```python
from build123d import *

# Parameters (mm, degrees)
HEX_START      = -10
SKETCH3_R      = 2
HEX_HEAD_DEPTH = 10


with BuildPart() as part:
    # Sketch1 → Main Base (revolve)
    with BuildSketch(Plane(origin=(0, 0, 0), x_dir=(0, 0, -1), z_dir=(1, 0, 0))):
        Polygon((0, 2), (0, 3), (-8.5, 3), (-8.5, 3.2), (-9.3, 4), (-14.2, 4), (-15, 3.2), (-17, 3.2), (-17, 5.9), (-18.6, 5.9), (-18.6, 7), (-28.6, 7), (-28.6, 2), align=None)
    revolve(axis=Axis((0, 0, -105.38083184), (0, 0, 1)))

    # Sketch3 → Hex Head (add)
    with BuildSketch(Plane.XY.offset(28.6).offset(HEX_START)):
        Polygon((8.082903769, 0), (4.041451884, 7), (-4.041451884, 7), (-8.082903769, 0), (-4.041451884, -7), (4.041451884, -7), align=None)
        with Locations(Location((0, 0, 0), (0, 0, 90))):
            Circle(SKETCH3_R, mode=Mode.SUBTRACT)
    extrude(amount=HEX_HEAD_DEPTH)

    # Sketch5 → Hex Trim (revolve, cut)
    with BuildSketch(Plane(origin=(0, 0, 0), x_dir=(1, 0, 0), z_dir=(0, 1, 0)), mode=Mode.PRIVATE) as hex_trim_sk:
        Polygon((-6.4, -18.6), (-7.5, -19.235085296), (-7.5, -27.964914704), (-6.4, -28.6), (-8.082903769, -28.6), (-8.082903769, -18.6), align=None)
    revolve(hex_trim_sk.sketch.rotate(Axis((0, 0, 20.51194439), (0, 0, 1)), 188.960530202), axis=Axis((0, 0, 20.51194439), (0, 0, 1)), mode=Mode.SUBTRACT)


solid = part.part
```
Design review of the part built by this model. Coordinates are the model's own, in mm. A direction names the side the tool comes from. Give positions to 0.01 mm unless a question says otherwise; leave off trailing zeros. Order: outer loops, then holes, each group sorted by start corner. A loop starts at its lowest first (then second) coordinate and runs counter-clockwise, first axis right, second up. Notation, with made-up numbers: (38, 33) -> (51, 33) arc R30 cw to (51, 58) -> close; hole circle Ø1 at (-24, -11.5). An arc over 180 degrees is marked (long way). Write item = value, one per line. Start each with the question number.
(1) For faces 4 (the face through (3, -3, 17)), 5 (the face through (-6.043, 3.533, 23.535)), 6 (the face through (0, -3, 4)), list the 3-axis set-ups (+Z, -Z, +X, -X, +Y, -Y) from which the entire face can be reached by the end or side of a thin tool; tool diameter is ignored.
(2) For pin 1 (1 mm diameter, centred on y = 0.5, z = 15, fed in from +X); pin 2 (3 mm diameter, centred on y = 3.5, z = 20, fed in from -X); pin 3 (2 mm diameter, centred on x = -4.5, z = 17, fed in from +Y), all flat-tipped, find the tip position at first contact; note any pin that passes through.
(3) To check wall thickness, follow line 1 along X through (y, z) = (0, 22.25); line 2 along X through (y, z) = (0, 11.25); line 3 along Y through (x, z) = (0, 7.75). State the ranges of each line that lie inside material, in increasing order.
(4) We need section C-C on z = 3. Write out the cut boundary in (x, y).
(5) We need section D-D on z = 12.5. Write out the cut boundary in (x, y), plus the area to 3 significant figures.
(6) Mouldability with a two-part tool opening along X and no side actions: class faces 1 (the face through (2, 0, 14)), 2 (the face through (3.74, -6.5, 23.66)), 3 (the face through (-0.259, -5.894, 17.811)) as +X half, -X half, draft (parallel to the pull), parting line (faces both ways), or undercut.
Numbers:
q1.face_4 = none
q1.face_5 = +Z, -Z, -X, +Y
q1.face_6 = -Z
q2.pin_1 = 3.67
q2.pin_2 = -6.93
q2.pin_3 = 4.75
q3.line_1 = -7.5 to -2, 2 to 7.5
q3.line_2 = -4 to -2, 2 to 4
q3.line_3 = -3 to -2, 2 to 3
q4.outline = circle Ø6 at (0, 0); hole circle Ø4 at (0, 0)
q5.outline = circle Ø8 at (0, 0); hole circle Ø4 at (0, 0)
q5.area = 37.7 mm^2
q6.face_1 = undercut
q6.face_2 = +X half
q6.face_3 = parting line
